Verification items for this drawing (mm, ordinates from the low corner). A direction names the side the tool comes from. Round coordinates to 2 decimals unless told otherwise and drop trailing zeros. Order: outer loops, then holes, each group sorted by start corner. A loop starts at its lowest first (then second) coordinate and runs counter-clockwise, first axis right, second up. Notation, with made-up numbers: (15, 19.5) -> (34, 19.5) arc R20 ccw to (34, 35.5) -> close; hole circle Ø7 at (60, 17). An arc over 180 degrees is marked (long way). Use a Markdown table: item, result. Add a question column.
Item 1: Mould release check, pull along X, two halves, no side actions. Record for the marked faces 1, 2 and 3: pulls with the +X half, pulls with the -X half, needs draft (parallel to the pull), parting line crosses it, or undercut.
Item 2: Material ranges on probe 1 along X at (y, z) = (9, 27.5); probe 2 along X at (y, z) = (58.5, 25); probe 3 along Y at (x, z) = (29, 34.5), recorded low to high. Write a range as [from, to].
Item 3: Sectioned sample at D-D, the plane y = 10.5. Record the cut outline in (x, z).
Item 4: Gauge pin test, flat ends, axial feed: pin 1 Ø6 at (x, z) = (76, 23.5) entering from -Y; pin 2 Ø12 at (y, z) = (40, 27.5) entering from -X; pin 3 Ø2 at (y, z) = (15.5, 34.5) entering from +X; pin 4 Ø9 at (x, z) = (15, 20.5) entering from +Y. Record the tip position at first contact, or that the pin passes through.
Item 5: Set-up check for the marked faces 4, 5, 6, 7 and 8: record each of +Z, -Z, +X, -X, +Y, -Y from which the full face is reachable in a straight line by a thin tool's end or side.
Item 6: Sectioned sample at C-C, the plane z = 33.5. Record the cut outline in (x, y).
Item 7: Sectioned sample at B-B, the plane x = 36.5. Record the cut outline in (y, z).
Item 8: Sectioned sample at A-A, the plane y = 25. Record the cut outline in (x, z).
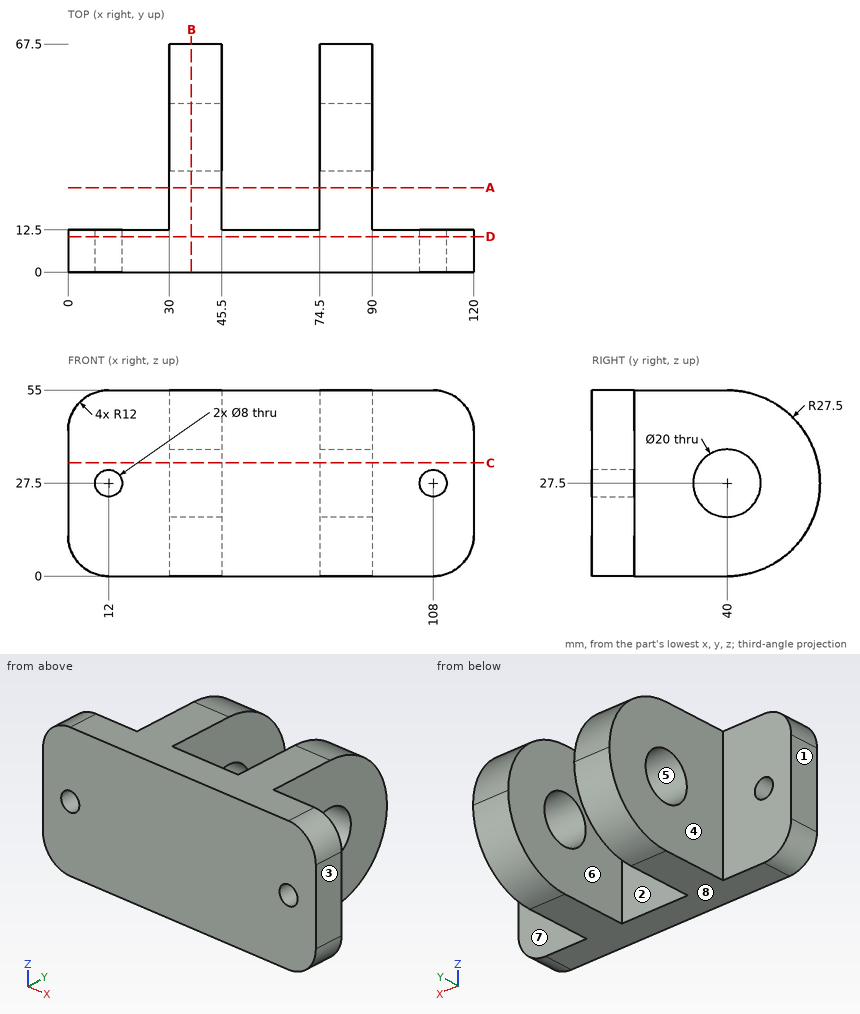
Found:
| question | item | result |
|---|---|---|
| 1 | face 1 | pulls with the -X half |
| 1 | face 2 | undercut |
| 1 | face 3 | pulls with the +X half |
| 2 | probe 1 | x = [0, 8], [16, 104], [112, 120] |
| 2 | probe 2 | x = [30, 45.5], [74.5, 90] |
| 2 | probe 3 | y = [0, 12.5] |
| 3 | outline | (0, 12) arc R12 ccw to (12, 0) -> (108, 0) arc R12 ccw to (120, 12) -> (120, 43) arc R12 ccw to (108, 55) -> (12, 55) arc R12 ccw to (0, 43) -> close; hole circle Ø8 at (12, 27.5); hole circle Ø8 at (108, 27.5) |
| 4 | pin 1 | stops at y = 0 |
| 4 | pin 2 | passes through |
| 4 | pin 3 | stops at x = 90 |
| 4 | pin 4 | stops at y = 12.5 |
| 5 | face 4 | +Z, -Z, -X, +Y |
| 5 | face 5 | +X, -X |
| 5 | face 6 | +Z, -Z, +Y |
| 5 | face 7 | +Z, -Z, +X, +Y |
| 5 | face 8 | -Z, +X, -X, +Y, -Y |
| 6 | outline | (0, 0) -> (120, 0) -> (120, 12.5) -> (90, 12.5) -> (90, 32) -> (74.5, 32) -> (74.5, 12.5) -> (45.5, 12.5) -> (45.5, 32) -> (30, 32) -> (30, 12.5) -> (0, 12.5) -> close; (30, 48) -> (45.5, 48) -> (45.5, 66.84) -> (30, 66.84) -> close; (74.5, 48) -> (90, 48) -> (90, 66.84) -> (74.5, 66.84) -> close |
| 7 | outline | (0, 0) -> (40, 0) arc R27.5 ccw to (40, 55) -> (0, 55) -> close; hole circle Ø20 at (40, 27.5) |
| 8 | outline | (30, 0) -> (45.5, 0) -> (45.5, 55) -> (30, 55) -> close; (74.5, 0) -> (90, 0) -> (90, 55) -> (74.5, 55) -> close |
